Part model, mm, in its own coordinate system. A direction names the side the tool comes from. Give positions to 0.01 mm unless a question says otherwise; leave off trailing zeros. Write each loop counter-clockwise with the first axis right and the second up, starting at its lowest first coordinate (ties: lowest second). Pieces come first, ordered by that corner, then holes.
from build123d import *

# Parameters (mm, degrees)
F0_R     = 1.25
F1_DEPTH = 5
F0_W     = 27
F0_H     = 50
F2_DEPTH = 1


with BuildPart() as f1:
    # F0 (on Top) → F1 (new body)
    with BuildSketch(Plane.XY):
        with Locations((-10.4, 21.85)):
            Circle(F0_R)
    extrude(amount=F1_DEPTH)



with BuildPart() as f1b:
    # F0 (on Top) → F1, piece 2 (new body)
    with BuildSketch(Plane.XY):
        with Locations((-10.4, -21.85)):
            Circle(F0_R)
    extrude(amount=F1_DEPTH)


with BuildPart() as f1c:
    # F0 (on Top) → F1, piece 3 (new body)
    with BuildSketch(Plane.XY):
        with Locations((10.4, -21.85)):
            Circle(F0_R)
    extrude(amount=F1_DEPTH)


with BuildPart() as f1d:
    # F0 (on Top) → F1, piece 4 (new body)
    with BuildSketch(Plane.XY):
        with Locations((10.4, 21.85)):
            Circle(F0_R)
    extrude(amount=F1_DEPTH)


with BuildPart() as f1_1:
    add(f1.part)

    add(f1b.part)  # F2 merges F1b

    add(f1c.part)  # F2 merges F1c

    add(f1d.part)  # F2 merges F1d
    # F0 (on Top) → F2 (join)
    with BuildSketch(Plane.XY):
        Rectangle(F0_W, F0_H)
        with Locations((-10.4, -21.85)):
            Circle(F0_R, mode=Mode.SUBTRACT)
        with Locations((10.4, -21.85)):
            Circle(F0_R, mode=Mode.SUBTRACT)
        with Locations((-10.4, 21.85)):
            Circle(F0_R, mode=Mode.SUBTRACT)
        with Locations((10.4, 21.85)):
            Circle(F0_R, mode=Mode.SUBTRACT)
    extrude(amount=F2_DEPTH)


solid = f1_1.part
1) Flat gauge pins, fed straight in: P1, Ø13.5, axis at x = -1, y = -12.5, coming from the +Z side; P2, Ø1, axis at x = -8.5, y = -5.5, coming from the -Z side; P3, Ø2, axis at x = -3.5, z = 2.5, coming from the -Y side. Where does each tip first touch, or does it go through?
Check result:
P1: stops at z = 1
P2: stops at z = 0
P3: passes through
2) Saw through at B-B (y = -21.85). Write the cut outline in (x, z).
Check result:
outline: (-13.5, 0) - (13.5, 0) - (13.5, 1) - (11.65, 1) - (11.65, 5) - (9.15, 5) - (9.15, 1) - (-9.15, 1) - (-9.15, 5) - (-11.65, 5) - (-11.65, 1) - (-13.5, 1) - close
3) Mould opens along Y. For faces 3 (the flat face through (-13.5, -0.3, 0.5)), 4 (the cylindrical face through (11.072, 22.904, 2.972)), 5 (the flat face through (-0.2, -25, 0.5)) say: +Y half, -Y half, draft (parallel to the pull), parting line (faces both ways), or undercut.
Check result:
face 3: draft
face 4: undercut
face 5: -Y half
4) Saw through at D-D (x = -6). Write the cut outline in (y, z).
Check result:
outline: (-25, 0) - (25, 0) - (25, 1) - (-25, 1) - close
5) Drill centre lines: L1, parallel to Z at x = 5.75, y = 1.5; L2, parallel to Y at x = -10.5, z = 4.6; L3, parallel to X at y = -21, z = 2.7. Where is each one in solid material? Low to high.
Check result:
L1: z = 0 to 1
L2: y = -23.1 to -20.6, 20.6 to 23.1
L3: x = -11.32 to -9.48, 9.48 to 11.32
6) 3-axis set-ups, long thin cutter, end or side, ignore diameter. For faces 1 (the cylindrical face through (-11.321, 22.695, 2.972)), 2 (the flat face through (10, 22, 5)): which of +Z, -Z, +X, -X, +Y, -Y reach the whole face in a straight line?
Check result:
face 1: +Z
face 2: +Z, +X, -X, +Y, -Y
7) Saw through at A-A (x = -10.4). Write the cut outline in (y, z).
Check result:
outline: (-25, 0) - (25, 0) - (25, 1) - (23.1, 1) - (23.1, 5) - (20.6, 5) - (20.6, 1) - (-20.6, 1) - (-20.6, 5) - (-23.1, 5) - (-23.1, 1) - (-25, 1) - close
8) Saw through at C-C (z = 3.3). Write the cut outline in (x, y).
Check result:
outline: circle Ø2.5 at (-10.4, -21.85); circle Ø2.5 at (-10.4, 21.85); circle Ø2.5 at (10.4, -21.85); circle Ø2.5 at (10.4, 21.85)
